Geometry: final body of the model. Coordinates: model frame, mm. Face numbers are marked on the shaded views. Coordinates: 2 decimals unless noted, no trailing zeros. Order: outer loops, then holes, each group sorted by start corner. A loop starts at its lowest first (then second) coordinate and runs counter-clockwise, first axis right, second up. Notation, with made-up numbers: (46.5, 74.25) - (84.5, 74.25) arc R10 ccw to (84.5, 84.25) - close; hole circle Ø5 at (-25.5, 73). An arc over 180 degrees is marked (long way). Use a Markdown table: item, result. Add a question column.
```python
from build123d import *

# Parameters (mm, degrees)
SKETCH1_R           = 1.5
BOSS_EXTRUDE1_DEPTH = 1.1
SKETCH2_W           = 3
SKETCH2_H           = 5.15
BOSS_EXTRUDE2_DEPTH = 1.1
SKETCH3_W           = 1.4
SKETCH3_H           = 3
CUT_EXTRUDE1_DEPTH  = 0.2


with BuildPart() as part:
    # Sketch1 → Boss-Extrude1 (new body)
    with BuildSketch(Plane(origin=(0, 0, 0), x_dir=(1, 0, 0), z_dir=(0, 1, 0))):
        with BuildLine():
            Line((-20, 4.5), (20, 4.5))
            ThreePointArc((20, 4.5), (21.767766953, 3.767766953), (22.5, 2))
            Line((22.5, 2), (22.5, -2))
            ThreePointArc((22.5, -2), (21.767766953, -3.767766953), (20, -4.5))
            Line((20, -4.5), (-20, -4.5))
            ThreePointArc((-20, -4.5), (-21.767766953, -3.767766953), (-22.5, -2))
            Line((-22.5, -2), (-22.5, 2))
            ThreePointArc((-22.5, 2), (-21.767766953, 3.767766953), (-20, 4.5))
        make_face()
        with Locations(Location((-19.5, 0, 0), (0, 0, 270))):
            Circle(SKETCH1_R, mode=Mode.SUBTRACT)
        with Locations(Location((19.5, 0, 0), (0, 0, 90))):
            Circle(SKETCH1_R, mode=Mode.SUBTRACT)
    extrude(amount=BOSS_EXTRUDE1_DEPTH)

    # Sketch2 → Boss-Extrude2 (add)
    with BuildSketch(Plane(origin=(0, 1.1, 0), x_dir=(1, 0, 0), z_dir=(0, 1, 0))):
        with Locations((15, 0)):
            Rectangle(SKETCH2_W, SKETCH2_H)
        with Locations((-15, 0)):
            Rectangle(SKETCH2_W, SKETCH2_H)
        Rectangle(SKETCH2_W, SKETCH2_H)
    extrude(amount=BOSS_EXTRUDE2_DEPTH)

    # Sketch3 → Cut-Extrude1 (cut)
    with BuildSketch(Plane(origin=(0, 2.2, 0), x_dir=(1, 0, 0), z_dir=(0, 1, 0))):
        with Locations((15, 0)):
            Rectangle(SKETCH3_W, SKETCH3_H)
        with Locations((-15, 0)):
            Rectangle(SKETCH3_W, SKETCH3_H)
        Rectangle(SKETCH3_W, SKETCH3_H)
    extrude(amount=-CUT_EXTRUDE1_DEPTH, mode=Mode.SUBTRACT)


solid = part.part
```
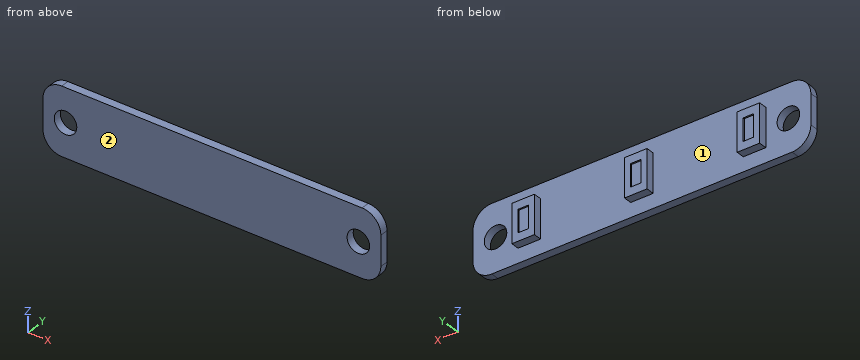
1) Draft query along X for the marked faces 1 and 2. Return one class per face: pulls with the +X half, pulls with the -X half, needs draft (parallel to the pull), parting line crosses it, or undercut.
2) Section C-C (x = -10.5). Return loops of the section in (y, z).
3) Section A-A (x = -19.5). Return loops of the section in (y, z), then the cut area to 3 significant figures.
4) Pin query (flat end, axial travel): pin 1 (0.9 mm diameter, centred on x = 14.5, y = 2, fed in from -Z) (3 decimals); pin 2 (0.9 mm diameter, centred on y = 1.5, z = 0.5, fed in from -X); pin 3 (2.5 mm diameter, centred on x = -19.5, z = 0, fed in from +Y); pin 4 (1 mm diameter, centred on x = 11, z = 3, fed in from +Y). Return the tip coordinate at first contact, or that it passes through.
5) Ray query, line 1 along X through (y, z) = (0.75, 0); line 2 along Z through (x, y) = (19.5, 0.55); line 3 along Y through (x, z) = (4.5, -2.75). Return the intervals inside material, ascending.
6) Section B-B (z = 0). Give the number of separate pieces and of enclosed holes in the cut face, then the cut area to 3 significant figures.
Values follow:
| question | item | result |
|---|---|---|
| 1 | face 1 | undercut |
| 1 | face 2 | needs draft |
| 2 | outline | (0, -4.5) - (1.1, -4.5) - (1.1, 4.5) - (0, 4.5) - close |
| 3 | outline | (0, -4.5) - (1.1, -4.5) - (1.1, -1.5) - (0, -1.5) - close; (0, 1.5) - (1.1, 1.5) - (1.1, 4.5) - (0, 4.5) - close |
| 3 | area | 6.60 mm² |
| 4 | pin 1 | stops at z = -2.575 |
| 4 | pin 2 | stops at x = -22.5 |
| 4 | pin 3 | passes through |
| 4 | pin 4 | stops at y = 1.1 |
| 5 | line 1 | x = -22.5 to -21, -18 to 18, 21 to 22.5 |
| 5 | line 2 | z = -4.5 to -1.5, 1.5 to 4.5 |
| 5 | line 3 | y = 0 to 1.1 |
| 6 | separate pieces | 3 |
| 6 | enclosed holes | 0 |
| 6 | area | 52.0 mm² |
